Work out the finished part from the listing and answer in its coordinate system (mm). Face numbers are marked on the shaded views. A direction names the side the tool comes from. Round coordinates to 2 decimals unless told otherwise and drop trailing zeros. Write each loop counter-clockwise with the first axis right and the second up, starting at its lowest first coordinate (ties: lowest second). Pieces come first, ordered by that corner, then holes. Notation, with made-up numbers: (20, 69) -> (69, 69) arc R21 ccw to (69, 97) -> close; hole circle Ø7 at (-11.5, -21). An arc over 180 degrees is marked (long way). One line per question, with ' | ' between items. Start each with the question number.
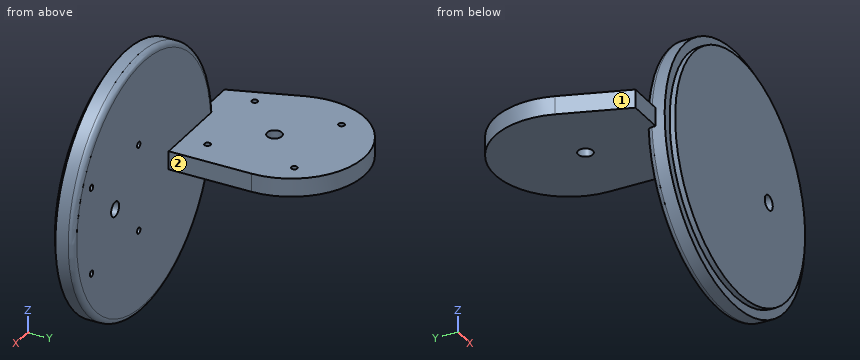
```python
from build123d import *

# Parameters (mm, degrees)
SKETCH1_R                 = 70
BOSS_EXTRUDE1_DEPTH       = 10
SKETCH2_R                 = 65
BOSS_EXTRUDE4_DEPTH       = 3
BOSS_EXTRUDE5_DEPTH       = 5
M4X0_7_TAPPED_HOLE1_D     = 3.3
M4X0_7_TAPPED_HOLE1_DEPTH = 6
M4X0_7_TAPPED_HOLE1_TIP   = 0.991420021
F_8_0MM_DOWEL_HOLE2_D     = 8
M4X0_7_TAPPED_HOLE3_D     = 3.3
M4X0_7_TAPPED_HOLE3_DEPTH = 6
M4X0_7_TAPPED_HOLE3_TIP   = 0.991420021
F_8_0MM_DOWEL_HOLE3_D     = 8
FILLET1_R                 = 3


with BuildPart() as part:
    # Sketch1 → Boss-Extrude1 (new body)
    with BuildSketch(Plane(origin=(0, 0, 0), x_dir=(1, 0, 0), z_dir=(0, 1, 0))):
        with Locations(Location((0, 0, 0), (0, 0, 270))):
            Circle(SKETCH1_R)
    extrude(amount=BOSS_EXTRUDE1_DEPTH)

    # Sketch2 → Boss-Extrude4 (add)
    with BuildSketch(Plane.XZ):
        with Locations(Location((0, 0, 0), (0, 0, 270))):
            Circle(SKETCH2_R)
    extrude(amount=BOSS_EXTRUDE4_DEPTH)

    # Sketch3 → Boss-Extrude5 (add, symmetric)
    with BuildSketch(Plane.XY):
        with BuildLine():
            Line((-25, 55), (-25, 5))
            Line((-25, 5), (-90, 5))
            Line((-90, 5), (-102.792798963, 41.896399481))
            ThreePointArc((-102.792798963, 41.896399481), (-71.644096684, 94.444340269), (-25, 55))
        make_face()
    extrude(amount=BOSS_EXTRUDE5_DEPTH, both=True)

    # M4x0.7 Tapped Hole1
    with Locations(Plane(origin=(0, 10, 0), x_dir=(1, 0, 0), z_dir=(0, 1, 0))):
        with Locations((5, 23.622), (52.244, 23.622), (52.244, -23.622), (5, -23.622)):
            Hole(M4X0_7_TAPPED_HOLE1_D / 2, depth=M4X0_7_TAPPED_HOLE1_DEPTH)
            with Locations((0, 0, -(M4X0_7_TAPPED_HOLE1_DEPTH + M4X0_7_TAPPED_HOLE1_TIP / 2))):  # 118° drill point
                Cone(0, M4X0_7_TAPPED_HOLE1_D / 2, M4X0_7_TAPPED_HOLE1_TIP, mode=Mode.SUBTRACT)

    # Ø8.0mm Dowel Hole2 (through all)
    with Locations(Plane(origin=(0, 0, -5), x_dir=(1, 0, 0), z_dir=(0, 0, -1))):
        with Locations((-63.420285579, -46.697024874)):
            Hole(F_8_0MM_DOWEL_HOLE2_D / 2)

    # M4x0.7 Tapped Hole3
    with Locations(Plane.XY.offset(5)):
        with Locations((-87.040285579, 70.317024874), (-39.800285579, 70.317024874), (-39.800285579, 23.077024874), (-87.040285579, 23.077024874)):
            Hole(M4X0_7_TAPPED_HOLE3_D / 2, depth=M4X0_7_TAPPED_HOLE3_DEPTH)
            with Locations((0, 0, -(M4X0_7_TAPPED_HOLE3_DEPTH + M4X0_7_TAPPED_HOLE3_TIP / 2))):  # 118° drill point
                Cone(0, M4X0_7_TAPPED_HOLE3_D / 2, M4X0_7_TAPPED_HOLE3_TIP, mode=Mode.SUBTRACT)

    # Ø8.0mm Dowel Hole3 (through all)
    with Locations(Plane(origin=(0, 10, 0), x_dir=(1, 0, 0), z_dir=(0, 1, 0))):
        with Locations((28.624, -0.002)):
            Hole(F_8_0MM_DOWEL_HOLE3_D / 2)

    # Fillet1
    fillet1_edges = [part.edges().sort_by_distance(p)[0] for p in [
        (51.23475383, 10, -47.696960071),
    ]]
    fillet(fillet1_edges, radius=FILLET1_R)


solid = part.part
```
(1) A cutting plane is placed at C-C, the plane y = 29.5. Determine the outline of the cut face in (x, z).
(2) Given pin 1 Ø5 at (x, z) = (28.624, 0.002) entering from -Y; pin 2 Ø4.5 at (x, z) = (52.244, -23.622) entering from +Y; pin 3 Ø10.5 at (x, y) = (-63.42, 46.7) entering from -Z; pin 4 Ø11 at (y, z) = (43, 1.5) entering from +X, each flat-ended and moving along its own axis, determine where each tip first touches the part or whether it passes through.
(3) For the marked faces 1 and 2, determine the directions among +Z, -Z, +X, -X, +Y, -Y from which every point of the face is accessible in a straight line to the end or side of a thin tool.
(4) A cutting plane is placed at A-A, the plane x = 0. Determine the outline of the cut face in (y, z), then the cut area to 3 significant figures.
(5) Consider L1, parallel to Y at x = 42, z = 11.5; L2, parallel to Z at x = -93.5, y = 19; L3, parallel to Y at x = 60, z = -29. Determine where each line is inside the solid, lowest interval first.
(6) A cutting plane is placed at B-B, the plane y = 74.5. Determine the outline of the cut face in (x, z).
Returned:
1) outline: (-98.49, -5) -> (-25, -5) -> (-25, 5) -> (-98.49, 5) -> close
2) pin 1: through | pin 2: y = 10 | pin 3: z = -5 | pin 4: x = -25
3) face 1: +Z, -Z, -X, -Y | face 2: +Z, -Z, +X, +Y
4) outline: (-3, -65) -> (0, -65) -> (0, -70) -> (7, -70) arc R3 ccw to (10, -67) -> (10, 67) arc R3 ccw to (7, 70) -> (0, 70) -> (0, 65) -> (-3, 65) -> close | area: 1,790 mm2
5) L1: -3 to 10 | L2: -5 to 5 | L3: 0 to 10
6) outline: (-99.92, -5) -> (-30.08, -5) -> (-30.08, 5) -> (-99.92, 5) -> close
